Check sheet for the drawn part. Datum: minimum x, y, z corner. Units: mm. A direction names the side the tool comes from. Round coordinates to 2 decimals unless told otherwise and drop trailing zeros. Order: outer loops, then holes, each group sorted by start corner. A loop starts at its lowest first (then second) coordinate and runs counter-clockwise, first axis right, second up. Notation, with made-up numbers: M 53,-27 L 69,-27 A13 cw 69,-21 Z; hole C 3,77 d8. An arc over 180 degrees is marked long. Use one line per item in the form item = value. Start each with the question number.
Item 1: Cross-section at C-C on y = 1.5. Enter the section's corners in (x, z).
Item 2: Release check for a two-part mould opening along Y. For the marked faces 1, 2 and 3 record: +Y half, -Y half, draft (parallel to the pull), parting line (faces both ways), or undercut.
Item 3: Go/stop test with a flat-tipped pin: pin 1 Ø2 at (x, z) = (8, 18) entering from -Y. Record where the tip stops, or that it passes through.
Item 4: Cross-section at A-A on x = 9.75. Enter the section's corners in (y, z).
Item 5: Cross-section at B-B on z = 12.75. Enter the section's corners in (x, y), then the cut area to 3 significant figures.
Item 6: Thickness scan on probe 1 along Y at (x, z) = (4.75, 5.25); probe 2 along X at (y, z) = (8.5, 17.75) (1 decimal); probe 3 along X at (y, z) = (7, 11.25) (1 decimal). Record the ranges inside material, lowest first. Write a range as [from, to].
Item 7: Cross-section at D-D on x = 3.5. Enter the section's corners in (y, z) (1 decimal).
Item 8: Tool access check on the marked faces 4 and 5. Record the directions out of +Z, -Z, +X, -X, +Y, -Y that give a thin tool (end or side, any length) a straight path to the whole face; none if there is none.
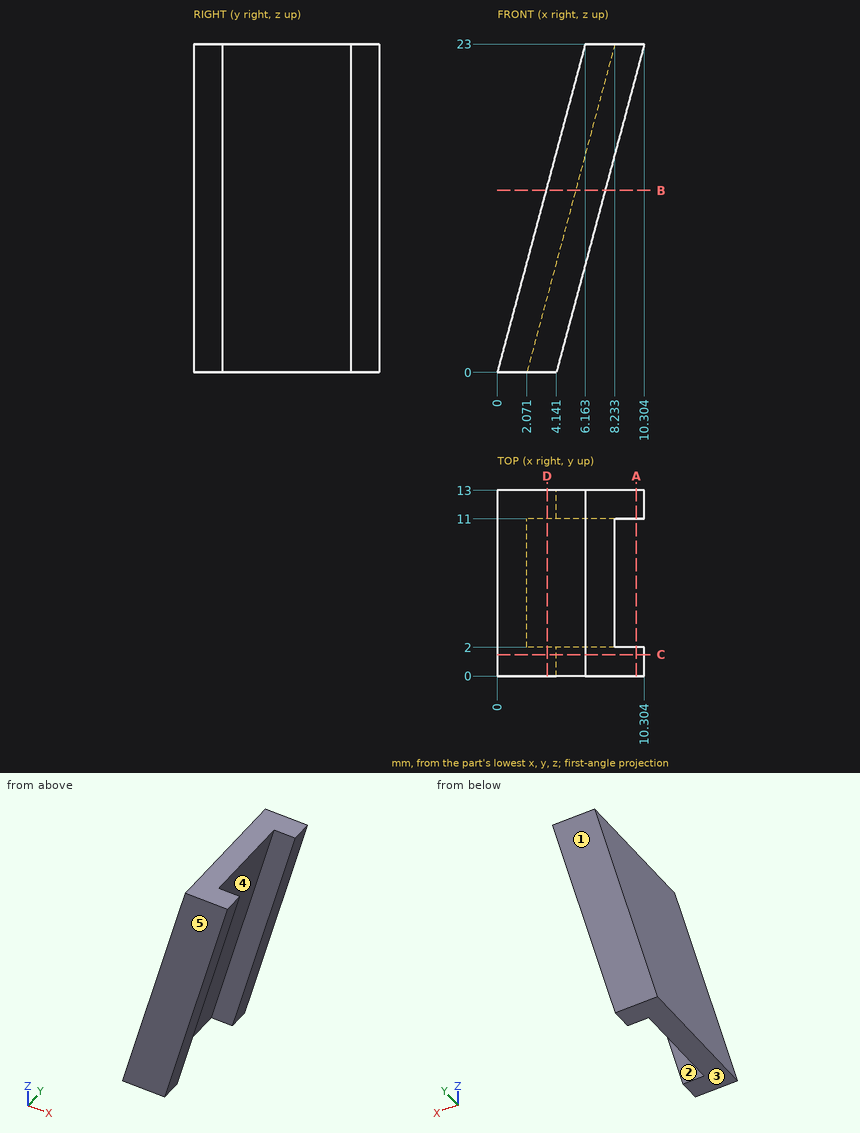
Output values:
q1.outline = M 0,0 L 4.14,0 L 10.3,23 L 6.16,23 Z
q2.face_1 = +Y half
q2.face_2 = undercut
q2.face_3 = draft
q3.pin_1 = 0
q4.outline = M 0,20.93 L 2,20.93 L 2,23 L 0,23 Z; M 11,20.93 L 13,20.93 L 13,23 L 11,23 Z
q5.outline = M 3.42,0 L 7.56,0 L 7.56,2 L 5.49,2 L 5.49,11 L 7.56,11 L 7.56,13 L 3.42,13 Z
q5.area = 35.2 mm2
q6.probe_1 = [0, 2], [11, 13]
q6.probe_2 = [4.8, 6.8]
q6.probe_3 = [3, 5.1]
q7.outline = M 0,0 L 2,0 L 2,5.3 L 11,5.3 L 11,0 L 13,0 L 13,13.1 L 0,13.1 Z
q8.face_4 = -Z, +X
q8.face_5 = +Z, -Z, +X, -X, -Y
